from build123d import *

# Parameters (mm, degrees)
BOSS_EXTRUDE1_DEPTH = 9.56
SKETCH2_R           = 2.45
BOSS_EXTRUDE2_DEPTH = 1.8
SHELL1_T            = -1.5
SKETCH3_R           = 1.48
BOSS_EXTRUDE4_DEPTH = 7.86


with BuildPart() as part:
    # Sketch1 → Boss-Extrude1 (new body)
    with BuildSketch(Plane(origin=(0, 0, 0), x_dir=(1, 0, 0), z_dir=(0, 1, 0))):
        Polygon((0, 0), (0, 7.89), (7.89, 7.89), (7.89, -7.89), (-7.89, -7.89), (-7.89, 0), align=None)
    extrude(amount=-BOSS_EXTRUDE1_DEPTH)

    # Sketch2 → Boss-Extrude2 (add)
    with BuildSketch(Plane(origin=(0, 0, 0), x_dir=(1, 0, 0), z_dir=(0, 1, 0))):
        with Locations(Location((3.945, -3.945, 0), (0, 0, 270))):
            Circle(SKETCH2_R)
        with Locations(Location((3.945, 3.955, 0), (0, 0, 270))):
            Circle(SKETCH2_R)
        with Locations(Location((-3.955, -3.945, 0), (0, 0, 270))):
            Circle(SKETCH2_R)
    extrude(amount=BOSS_EXTRUDE2_DEPTH)

    # Shell1
    shell1_openings = [part.faces().sort_by_distance(p)[0] for p in [
        (1.315, -9.56, 1.315),
    ]]
    offset(amount=SHELL1_T, openings=shell1_openings, kind=Kind.INTERSECTION)

    # Sketch3 → Boss-Extrude4 (add)
    with BuildSketch(Plane.XZ.offset(1.5)):
        with Locations(Location((0, 3.945, 0), (0, 0, 90))):
            Circle(SKETCH3_R)
        with Locations(Location((3.945, 0, 0), (0, 0, 90))):
            Circle(SKETCH3_R)
    extrude(amount=BOSS_EXTRUDE4_DEPTH)


solid = part.part
Design review of the part built by this model. Coordinates are the model's own, in mm. A direction names the side the tool comes from. Coordinates: 2 decimals unless noted, no trailing zeros. Write each loop counter-clockwise with the first axis right and the second up, starting at its lowest first coordinate (ties: lowest second). Pieces come first, ordered by that corner, then holes. Notation, with made-up numbers: (63, 16) - (69, 16) arc R21 ccw to (69, 51) - close; hole circle Ø4 at (59.5, -35.75). An arc over 180 degrees is marked (long way). One line per item, written item: value.
1) Insertion check: pin 1 (1.5 mm diameter, centred on x = 4, z = 3.5, fed in from -Y); pin 2 (2.5 mm diameter, centred on y = -4, z = -4.5, fed in from -X); pin 3 (0.9 mm diameter, centred on x = 0.5, z = 4, fed in from -Y). Each pin has a flat end and moves straight along its axis. Give the tip position at first contact, or say it passes through.
Answer sheet:
pin 1: stops at y = -1.5
pin 2: stops at x = 0
pin 3: stops at y = -9.36
2) For faces 1 (the face through (4, 1.8, -4)), 2 (the face through (6.39, -5, 0)), 3 (the face through (0, -5, 7.89)), 4 (the face through (4.681, 0.887, 6.282)), 5 (the face through (-4, -5, 0)), list the 3-axis set-ups (+Z, -Z, +X, -X, +Y, -Y) from which the entire face can be reached by the end or side of a thin tool; tool diameter is ignored.
Answer sheet:
face 1: +Z, -Z, +X, -X, +Y
face 2: -Y
face 3: +Z, +X, -X, +Y, -Y
face 4: +Y
face 5: -Z, -X, +Y, -Y
3) Add section A-A (y = -4.5). State the section outline as (x, z) points (3 decimals).
Answer sheet:
outline: (-7.89, 0) - (0, 0) - (0, -7.89) - (7.89, -7.89) - (7.89, 7.89) - (-7.89, 7.89) - close; circle Ø2.96 at (0, 3.945); circle Ø2.96 at (3.945, 0); hole (-6.39, 1.5) - (1.5, 1.5) - (1.5, -6.39) - (6.39, -6.39) - (6.39, 6.39) - (-6.39, 6.39) - close
4) To check wall thickness, follow probe 1 along X at (y, z) = (-6.25, -2.5); probe 2 along X at (y, z) = (-0.75, -4). State the ranges of each line that lie inside material, in increasing order.
Answer sheet:
probe 1: x = 0 to 1.5, 6.39 to 7.89
probe 2: x = 0 to 3, 4.89 to 7.89
5) Add section C-C (x = 4.25). State the section outline as (y, z) points, plus the area to 3 significant figures.
Answer sheet:
outline: (-9.56, -7.89) - (0, -7.89) - (0, -6.39) - (1.8, -6.39) - (1.8, -1.52) - (0, -1.52) - (0, 1.51) - (1.8, 1.51) - (1.8, 6.38) - (0, 6.38) - (0, 7.89) - (-9.56, 7.89) - (-9.56, 6.39) - (-1.5, 6.39) - (-1.5, 4.84) - (0.3, 4.84) - (0.3, 3.05) - (-1.5, 3.05) - (-1.5, 1.45) - (-9.36, 1.45) - (-9.36, -1.45) - (-1.5, -1.45) - (-1.5, -3.06) - (0.3, -3.06) - (0.3, -4.85) - (-1.5, -4.85) - (-1.5, -6.39) - (-9.56, -6.39) - close
area: 81.6 mm2
6) Mouldability with a two-part tool opening along X and no side actions: class faces 6 (the face through (2, 0, 2)), 7 (the face through (4, -9.36, 0)), 8 (the face through (2.454, 0.887, -5.899)), 9 (the face through (1, -9.56, 1)) as +X half, -X half, draft (parallel to the pull), parting line (faces both ways), or undercut.
Answer sheet:
face 6: undercut
face 7: undercut
face 8: parting line
face 9: draft
7) Add section D-D (y = -1). State the section outline as (x, z) points (3 decimals), plus the area to 3 significant figures.
Answer sheet:
outline: (-7.89, 0) - (0, 0) - (0, -7.89) - (7.89, -7.89) - (7.89, 7.89) - (-7.89, 7.89) - close; hole circle Ø1.9 at (-3.955, 3.945); hole circle Ø1.9 at (3.945, -3.955); hole circle Ø1.9 at (3.945, 3.945)
area: 178 mm2
8) Add section B-B (z = -2.5). State the section outline as (x, y) points, plus the area to 3 significant figures.
Answer sheet:
outline: (0, -9.56) - (1.5, -9.56) - (1.5, -1.5) - (6.39, -1.5) - (6.39, -9.56) - (7.89, -9.56) - (7.89, 0) - (5.92, 0) - (5.92, 1.8) - (1.97, 1.8) - (1.97, 0) - (0, 0) - close
area: 43.1 mm2
